Build history of the part. All positions in model axes, mm. Round coordinates to 2 decimals unless told otherwise and drop trailing zeros.
Item 1: Band-saw the part on A-A, the plane z = 91. Count the separate pieces of the cut face and the enclosed holes in it, then the cut area to 3 significant figures.
Item 2: Drop flat-ended pins along their axis: pin 1 Ø5 at (y, z) = (30.5, -124.5) entering from -X; pin 2 Ø12 at (x, y) = (-148, 13.5) entering from -Z; pin 3 Ø5 at (y, z) = (8, 92.5) entering from +X. Give the stop position or say it passes through.
Item 3: Wall check: probe 1 along X at (y, z) = (31, 67); probe 2 along X at (y, z) = (43.5, 60); probe 3 along X at (y, z) = (21.5, 46). Give the ranges that are in metal, low to high.
```python
from build123d import *

# Parameters (mm, degrees)
BOSS_EXTRUDE1_DEPTH     = 50.8
CUT_EXTRUDE1_DEPTH      = 260.287236955
CUT_EXTRUDE1_DEPTH_BACK = 260.287236955
SKETCH6_RX              = 78.834045808
SKETCH6_RY              = 63.772521642


with BuildPart() as part:
    # Sketch3 → Boss-Extrude1 (new body)
    with BuildSketch(Plane(origin=(0, 0, 0), x_dir=(1, 0, 0), z_dir=(0, 1, 0))):
        with BuildLine():
            add(Edge.make_bspline(
                [(-190.5, 0), (-184.392726562, 37.537038237), (-157.261289847, 93.964093485), (-82.387478202, 146.622658841), (-31.311374143, 160.799884185), (0, 159.189909928)],
                knots=[0, 0, 0, 0, 0.424401366, 0.656369581, 1, 1, 1, 1], degree=3))
            add(Edge.make_bspline(
                [(190.5, 0), (184.392726562, 37.537038237), (157.261289847, 93.964093485), (82.387478202, 146.622658841), (31.311374143, 160.799884185), (0, 159.189909928)],
                knots=[0, 0, 0, 0, 0.424401366, 0.656369581, 1, 1, 1, 1], degree=3))
            add(Edge.make_bspline(
                [(190.5, 0), (192.064011793, -4.963501926), (201.967167766, -83.314618311), (174.696602041, -109.289958804), (151.630121659, -100.567984898), (131.410771519, -87.719783961), (96.843567628, -85.375403377), (78.692510144, -86.25882742), (58.833533072, -96.87938247), (37.30593461, -109.935798162), (21.349613946, -139.114767457), (0, -140.530090072)],
                knots=[0, 0, 0, 0, 0.166997052, 0.292320514, 0.319633117, 0.42673531, 0.45891405, 0.609241775, 0.641909704, 0.76680237, 1, 1, 1, 1], degree=3))
            add(Edge.make_bspline(
                [(-190.5, 0), (-192.064011793, -4.963501926), (-201.967167766, -83.314618311), (-174.696602041, -109.289958804), (-151.630121659, -100.567984898), (-131.410771519, -87.719783961), (-96.843567628, -85.375403377), (-78.692510144, -86.25882742), (-58.833533072, -96.87938247), (-37.30593461, -109.935798162), (-21.349613946, -139.114767457), (0, -140.530090072)],
                knots=[0, 0, 0, 0, 0.166997052, 0.292320514, 0.319633117, 0.42673531, 0.45891405, 0.609241775, 0.641909704, 0.76680237, 1, 1, 1, 1], degree=3))
        make_face()
    extrude(amount=BOSS_EXTRUDE1_DEPTH)

    # Sketch6 → Cut-Extrude1 (cut, two sides: drawn at the far end of the back side and taken through both)
    with BuildSketch(Plane(origin=(0, 24.086508497, 9.976958489), x_dir=(-1, 0, 0), z_dir=(0, 0.5000000000000041, -0.8660254037844364)).offset(-CUT_EXTRUDE1_DEPTH_BACK)):
        with Locations(Location((-106.808169671, 81.026464977), (0, 0, -180))):
            Ellipse(SKETCH6_RX, SKETCH6_RY)
        with Locations(Location((106.808169671, 81.026464977), (0, 0, 180))):
            Ellipse(SKETCH6_RX, SKETCH6_RY)
    extrude(amount=CUT_EXTRUDE1_DEPTH + CUT_EXTRUDE1_DEPTH_BACK, mode=Mode.SUBTRACT)


solid = part.part
```
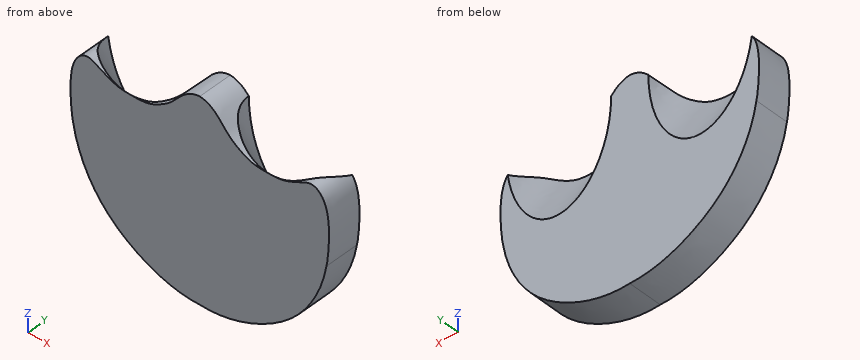
Results:
1. separate pieces: 3
1. enclosed holes: 0
1. area: 7,100 mm2
2. pin 1: stops at x = -115.95
2. pin 2: stops at z = -99.4
2. pin 3: stops at x = 187.65
3. probe 1: x = -193.52 to -160.72, -52.89 to 52.89, 160.72 to 193.52
3. probe 2: x = -194.12 to -168.99, -44.63 to 44.63, 168.99 to 194.12
3. probe 3: x = -194.5 to 194.5
